Job drawing, mm, ordinate dimensions from the low corner. One solid piece. Give positions to 0.01 mm unless a question says otherwise; leave off trailing zeros. Order: outer loops, then holes, each group sorted by start corner. A loop starts at its lowest first (then second) coordinate and runs counter-clockwise, first axis right, second up. Notation, with made-up numbers: (28.5, -27.75) -> (55.5, -27.75) arc R24 ccw to (55.5, -9.75) -> close; hole circle Ø5 at (78.5, 8). An arc over 180 degrees is marked (long way). Use CSV: the item, a comma, the result in double quotes. Start each with the question number.
1. Cut at B-B on z = 14.75. List the corners of the cut face in (x, y), then the cut area to 3 significant figures.
2. Wall check: line 1 (Y direction, x = 55, z = 10.5); line 2 (X direction, y = 53.5, z = 10); line 3 (X direction, y = 151, z = 1.75). Give the ranges that are in metal, low to high. Write a range as from..to.
3. Cut at A-A on y = 110. List the corners of the cut face in (x, z), then the cut area to 3 significant figures.
4. Cut at C-C on x = 55. List the corners of the cut face in (y, z).
5. Cut at D-D on y = 78.5. List the corners of the cut face in (x, z), then the cut area to 3 significant figures.
6. Pull direction X, two halves, no side cores. Call the marked faces 1, 2, 3 and 4: released by +X, released by -X, zero draft, split by the parting line, or undercut.
7. Drop flat-ended pins along their axis: pin 1 (3 mm diameter, centred on x = 95, z = 10, fed in from -Y); pin 2 (4 mm diameter, centred on y = 181, z = 13.5, fed in from -X); pin 3 (3 mm diameter, centred on x = 14.5, z = 11, fed in from +Y). Give the stop position or say it passes through.
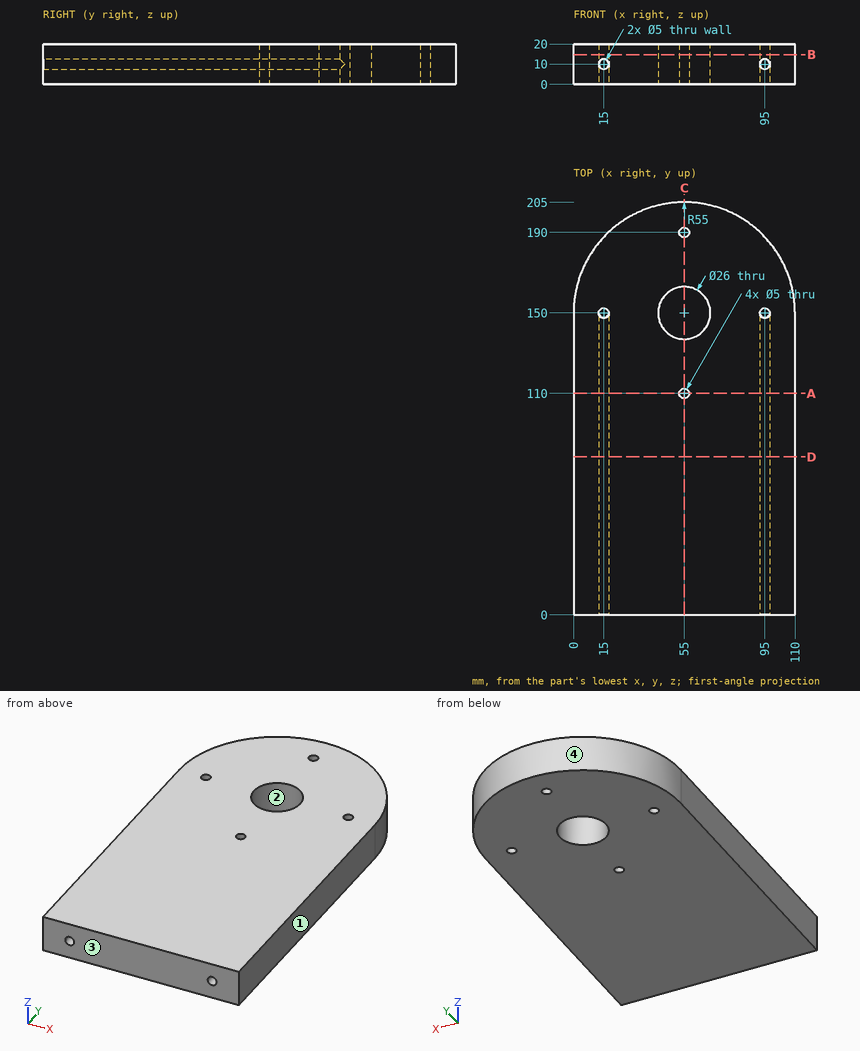
Verdict:
1,outline,"(0, 0) -> (110, 0) -> (110, 150) arc R55 ccw to (0, 150) -> close; hole circle Ø5 at (15, 150); hole circle Ø26 at (55, 150); hole circle Ø5 at (55, 110); hole circle Ø5 at (55, 190); hole circle Ø5 at (95, 150)"
1,area,"20,600 mm^2"
2,line 1,"0..107.5, 112.5..137, 163..187.5, 192.5..205"
2,line 2,"0..12.5, 17.5..92.5, 97.5..110"
2,line 3,"0.01..12.71, 17.29..42.04, 67.96..92.71, 97.29..109.99"
3,outline,"(0, 0) -> (52.5, 0) -> (52.5, 20) -> (0, 20) -> close; (57.5, 0) -> (110, 0) -> (110, 20) -> (57.5, 20) -> close; hole circle Ø5 at (15, 10); hole circle Ø5 at (95, 10)"
3,area,"2,060 mm^2"
4,outline,"(0, 0) -> (107.5, 0) -> (107.5, 20) -> (0, 20) -> close; (112.5, 0) -> (137, 0) -> (137, 20) -> (112.5, 20) -> close; (163, 0) -> (187.5, 0) -> (187.5, 20) -> (163, 20) -> close; (192.5, 0) -> (205, 0) -> (205, 20) -> (192.5, 20) -> close"
5,outline,"(0, 0) -> (110, 0) -> (110, 20) -> (0, 20) -> close; hole circle Ø5 at (15, 10); hole circle Ø5 at (95, 10)"
5,area,"2,160 mm^2"
6,face 1,"released by +X"
6,face 2,"undercut"
6,face 3,"zero draft"
6,face 4,"split by the parting line"
7,pin 1,"y = 152"
7,pin 2,"x = 8.27"
7,pin 3,"y = 188.78"
